Verification items for the finished model (mm, model axes). A direction names the side the tool comes from. Round coordinates to 2 decimals unless told otherwise and drop trailing zeros. Write each loop counter-clockwise with the first axis right and the second up, starting at its lowest first coordinate (ties: lowest second). Pieces come first, ordered by that corner, then holes. Notation, with made-up numbers: M 21.25,-9.5 L 29.25,-9.5 A8 ccw 29.25,3.5 Z; hole C 72.25,85.25 d2. An arc over 180 degrees is marked long. One line per item, written item: value. Start each with the question number.
from build123d import *

# Parameters (mm, degrees)
SKETCH1_R           = 3.3
BOSS_EXTRUDE1_DEPTH = 4
SKETCH2_W           = 19
SKETCH2_H           = 4
BOSS_EXTRUDE2_DEPTH = 18
SKETCH3_R           = 4.5
CUT_EXTRUDE1_DEPTH  = 4


with BuildPart() as part:
    # Sketch1 → Boss-Extrude1 (new body)
    with BuildSketch(Plane(origin=(0, 0, 0), x_dir=(1, 0, 0), z_dir=(0, 1, 0))):
        Polygon((0, 0), (25, 0), (25, 59), (45.5, 59), (45.5, 90), (0, 90), align=None)
        with Locations(Location((33.5, 71.5, 0), (0, 0, 270))):
            Circle(SKETCH1_R, mode=Mode.SUBTRACT)
        with Locations(Location((12.5, 12.5, 0), (0, 0, 270))):
            Circle(SKETCH1_R, mode=Mode.SUBTRACT)
    extrude(amount=BOSS_EXTRUDE1_DEPTH)

    # Sketch2 → Boss-Extrude2 (add)
    with BuildSketch(Plane(origin=(0, 4, 0), x_dir=(1, 0, 0), z_dir=(0, 1, 0))):
        with Locations((36, 88)):
            Rectangle(SKETCH2_W, SKETCH2_H)
    extrude(amount=BOSS_EXTRUDE2_DEPTH)

    # Sketch3 → Cut-Extrude1 (cut)
    with BuildSketch(Plane(origin=(0, 0, -90), x_dir=(-1, 0, 0), z_dir=(0, 0, -1))):
        with Locations((-36, 12.5)):
            Circle(SKETCH3_R)
    extrude(amount=-CUT_EXTRUDE1_DEPTH, mode=Mode.SUBTRACT)


solid = part.part
1) Thickness scan on line 1 (X direction, y = 3.1, z = -71.5); line 2 (Y direction, x = 36, z = -87); line 3 (Y direction, x = 23, z = -54.5). Record the ranges inside material, lowest first.
2) Cross-section at A-A (z = -71.5). Record the boundary of the cut face in (x, y).
3) Mould release check, pull along Z, two halves, no side actions. Record for faces 1 (the flat face through (26.5, 13, -88)), 2 (the cylindrical face through (33.6, 2, -74.8)), 3 (the flat face through (12, 2, 0)): pulls with the +Z half, pulls with the -Z half, needs draft (parallel to the pull), parting line crosses it, or undercut.
4) Cross-section at C-C (y = 12.5). Record the boundary of the cut face in (x, z).
5) Access from +Z, -Z, +X, -X, +Y, -Y to the whole of each face (thin tool, end or side, straight path). Record for faces 4 (the flat face through (25, 2, -29)), 5 (the flat face through (36, 22, -88)), 6 (the flat face through (34, 17, -86)).
6) Cross-section at D-D (x = 33.5). Record the boundary of the cut face in (y, z), then the cut area to 3 significant figures.
7) Gauge pin test, flat ends, axial feed: pin 1 Ø3 at (y, z) = (2, -32) entering from +X; pin 2 Ø6 at (x, z) = (17.5, -16) entering from +Y; pin 3 Ø1.2 at (x, y) = (37.5, 2) entering from +Z. Record the tip position at first contact, or that the pin passes through.
8) Cross-section at B-B (y = 2.5). Record the boundary of the cut face in (x, z), then the cut area to 3 significant figures.
Results below:
1. line 1: x = 0 to 30.2, 36.8 to 45.5
1. line 2: y = 0 to 8, 17 to 22
1. line 3: y = 0 to 4
2. outline: M 0,0 L 30.2,0 L 30.2,4 L 0,4 Z; M 36.8,0 L 45.5,0 L 45.5,4 L 36.8,4 Z
3. face 1: needs draft
3. face 2: undercut
3. face 3: pulls with the +Z half
4. outline: M 26.5,-90 L 31.5,-90 L 31.5,-86 L 26.5,-86 Z; M 40.5,-90 L 45.5,-90 L 45.5,-86 L 40.5,-86 Z
5. face 4: +Z, +X, +Y, -Y
5. face 5: +Z, -Z, +X, -X, +Y
5. face 6: +Z, +X, -X, +Y
6. outline: M 0,-90 L 8.76,-90 L 8.76,-86 L 4,-86 L 4,-74.8 L 0,-74.8 Z; M 0,-68.2 L 4,-68.2 L 4,-59 L 0,-59 Z; M 16.24,-90 L 22,-90 L 22,-86 L 16.24,-86 Z
6. area: 140 mm²
7. pin 1: stops at x = 25
7. pin 2: stops at y = 4
7. pin 3: stops at z = -59
8. outline: M 0,-90 L 45.5,-90 L 45.5,-59 L 25,-59 L 25,0 L 0,0 Z; hole C 12.5,-12.5 d6.6; hole C 33.5,-71.5 d6.6
8. area: 2,820 mm²
